from build123d import *

# Parameters (mm, degrees)
BOSS_EXTRUDE1_DEPTH = 65
CHAMFER1_SIZE       = 5
SKETCH4_R           = 23.5
SKETCH4_R_2         = 1.9
CUT_EXTRUDE1_DEPTH  = 65


with BuildPart() as part:
    # Sketch2 → Boss-Extrude1 (new body)
    with BuildSketch(Plane(origin=(0, 0, 0), x_dir=(0, 0, -1), z_dir=(1, 0, 0))):
        Polygon((0, 0), (0, 65), (-7, 65), (-7, -4), (65, -4), (65, 0), align=None)
    extrude(amount=BOSS_EXTRUDE1_DEPTH)

    # Chamfer1
    chamfer1_edges = [part.edges().sort_by_distance(p)[0] for p in [
        (65, 65, 3.5),
        (0, 65, 3.5),
    ]]
    chamfer(chamfer1_edges, length=CHAMFER1_SIZE)

    # Sketch4 → Cut-Extrude1 (cut)
    with BuildSketch(Plane.XY.offset(7)):
        with Locations((32.5, 30)):
            Circle(SKETCH4_R)
        with Locations((10, 52.5)):
            Circle(SKETCH4_R_2)
        with Locations((55, 52.5)):
            Circle(SKETCH4_R_2)
        with Locations((55, 7.5)):
            Circle(SKETCH4_R_2)
        with Locations((10, 7.5)):
            Circle(SKETCH4_R_2)
    extrude(amount=-CUT_EXTRUDE1_DEPTH, mode=Mode.SUBTRACT)


solid = part.part
Work out the finished part from the listing and answer in its coordinate system (mm). A direction names the side the tool comes from. Round coordinates to 2 decimals unless told otherwise and drop trailing zeros. Write each loop counter-clockwise with the first axis right and the second up, starting at its lowest first coordinate (ties: lowest second). Pieces come first, ordered by that corner, then holes.
1) A cutting plane is placed at D-D (y = 40). Give the vertices of the cut face in (x, z), plus the area to 3 significant figures.
2) The mould has two halves that part along X. Classify faces 3 (the flat face through (63, 62, 3)), 4 (the cylindrical face through (15.18, 45.88, 3.55)), 5 (the flat face through (32, 0, -33)): pulls with the +X half, pulls with the -X half, needs draft (parallel to the pull), parting line crosses it, or undercut.
3) A cutting plane is placed at C-C (x = 55). Give the vertices of the cut face in (y, z), plus the area to 3 significant figures.
4) A tool of negligible diameter and unlimited length cuts with its end or side. For faces 1 (the cylindrical face through (11.755, 6.772, 3.549)), 2 (the flat face through (32, 54, 0)), from which of +Z, -Z, +X, -X, +Y, -Y can it reach the whole face along a straight path? Write none if from no direction.
5) A cutting plane is placed at B-B (y = 30). Give the vertices of the cut face in (x, z), plus the area to 3 significant figures.
6) A cutting plane is placed at A-A (x = 32.5). Give the vertices of the cut face in (y, z), plus the area to 3 significant figures.
7) Straight lines are drawn through the part: line 1 (Y direction, x = 32.5, z = 2.5); line 2 (Y direction, x = 61, z = -49); line 3 (Z direction, x = 14, y = 62.5). For each, find the intervals that lie inside material, in ascending order.
8) Given pin 1 Ø2 at (x, z) = (28, -36) entering from +Y; pin 2 Ø4.5 at (x, y) = (10, 7.5) entering from -Z; pin 3 Ø3 at (x, y) = (55, 7.5) entering from +Z, each flat-ended and moving along its own axis, determine where each tip first touches the part or whether it passes through.
Completed:
1. outline: (0, 0) - (11.23, 0) - (11.23, 7) - (0, 7) - close; (53.77, 0) - (65, 0) - (65, 7) - (53.77, 7) - close
1. area: 157 mm2
2. face 3: pulls with the +X half
2. face 4: undercut
2. face 5: needs draft
3. outline: (-4, -65) - (0, -65) - (0, 0) - (5.6, 0) - (5.6, 7) - (-4, 7) - close; (9.4, 0) - (23.22, 0) - (23.22, 7) - (9.4, 7) - close; (36.78, 0) - (50.6, 0) - (50.6, 7) - (36.78, 7) - close; (54.4, 0) - (65, 0) - (65, 7) - (54.4, 7) - close
3. area: 595 mm2
4. face 1: +Z, -Z
4. face 2: -Z, +X, -X, +Y
5. outline: (0, 0) - (9, 0) - (9, 7) - (0, 7) - close; (56, 0) - (65, 0) - (65, 7) - (56, 7) - close
5. area: 126 mm2
6. outline: (-4, -65) - (0, -65) - (0, 0) - (6.5, 0) - (6.5, 7) - (-4, 7) - close; (53.5, 0) - (65, 0) - (65, 7) - (53.5, 7) - close
6. area: 414 mm2
7. line 1: y = -4 to 6.5, 53.5 to 65
7. line 2: y = -4 to 0
7. line 3: z = 0 to 7
8. pin 1: stops at y = 0
8. pin 2: stops at z = 0
8. pin 3: passes through
